Input: part model. Units: mm. Frame: model coordinates. Coordinates: 2 decimals unless noted, no trailing zeros. Loops run counter-clockwise (first coordinate to the right, second up) from the corner with the lowest first, then second, coordinate; pieces in that order, holes last. Notation, with made-up numbers: (8, 58) - (25, 58) arc R34 cw to (25, 90) - close; hole circle Ø2 at (-28, 66.5). An arc over 180 degrees is marked (long way). Use one line per item in the form item = value.
from build123d import *

# Parameters (mm, degrees)
EXTRU_MINCE1_DEPTH = 24


with BuildPart() as part:
    # Esquisse1 → Extru.-Mince1 (new body, symmetric)
    with BuildSketch(Plane.XY):
        with BuildLine():
            Line((547.565725672, -0.87294791), (541.301863245, 18.120841272))
            ThreePointArc((541.301863245, 18.120841272), (542.138161234, 23.516038085), (547, 26))
            ThreePointArc((547, 26), (551.756047412, 23.65787001), (552.799001066, 18.460004337))
            Line((552.799001066, 18.460004337), (547.665682189, -0.869999215))
            Line((547.665682189, -0.869999215), (550, -80))
            Line((550, -80), (550, -1562))
            ThreePointArc((550, -1562), (547.656854249, -1567.656854249), (542, -1570))
            Line((542, -1570), (-542, -1570))
            ThreePointArc((-542, -1570), (-547.656854249, -1567.656854249), (-550, -1562))
            Line((-550, -1562), (-550, -80))
            Line((-550, -80), (-547.665682189, -0.869999215))
            Line((-547.665682189, -0.869999215), (-552.799001066, 18.460004337))
            ThreePointArc((-552.799001066, 18.460004337), (-551.756047412, 23.65787001), (-547, 26))
            ThreePointArc((-547, 26), (-542.138161234, 23.516038085), (-541.301863245, 18.120841272))
            Line((-541.301863245, 18.120841272), (-547.565725672, -0.87294791))
            Line((-547.565725672, -0.87294791), (-544.716657295, -1.812527274))
            Line((-544.716657295, -1.812527274), (-538.452794868, 17.181261908))
            ThreePointArc((-538.452794868, 17.181261908), (-539.707241851, 25.274057128), (-547, 29))
            ThreePointArc((-547, 29), (-554.134071119, 25.486805015), (-555.698501598, 17.690006505))
            Line((-555.698501598, 17.690006505), (-550.677252807, -1.217986412))
            Line((-550.677252807, -1.217986412), (-553, -79.955759949))
            Line((-553, -79.955759949), (-553, -1562))
            ThreePointArc((-553, -1562), (-549.778174593, -1569.778174593), (-542, -1573))
            Line((-542, -1573), (542, -1573))
            ThreePointArc((542, -1573), (549.778174593, -1569.778174593), (553, -1562))
            Line((553, -1562), (553, -79.955759949))
            Line((553, -79.955759949), (550.677252807, -1.217986412))
            Line((550.677252807, -1.217986412), (555.698501598, 17.690006505))
            ThreePointArc((555.698501598, 17.690006505), (554.134071119, 25.486805015), (547, 29))
            ThreePointArc((547, 29), (539.707241851, 25.274057128), (538.452794868, 17.181261908))
            Line((538.452794868, 17.181261908), (544.716657295, -1.812527274))
            Line((544.716657295, -1.812527274), (547.565725672, -0.87294791))
        make_face()
    extrude(amount=EXTRU_MINCE1_DEPTH, both=True)


solid = part.part
Q1. Cut plane A-A, the plane y = -569. Return loops of the section in (x, z), then the cut area to 3 significant figures.
Check values:
outline = (-553, -24) - (-550, -24) - (-550, 24) - (-553, 24) - close; (550, -24) - (553, -24) - (553, 24) - (550, 24) - close
area = 288 mm²
Q2. Ray query, line 1 along X through (y, z) = (20, 9); line 2 along X through (y, z) = (-357, 6.5); line 3 along Y through (x, z) = (-143, -18.5). Return the intervals inside material, ascending. Write a range as [from, to].
Check values:
line_1 = [-556, -553], [-541, -538], [538, 541], [553, 556]
line_2 = [-553, -550], [550, 553]
line_3 = [-1573, -1570]
Q3. Pull-direction query (X, two-part tool) for faces 1 (the flat face through (-8, -1573, 0)), 2 (the flat face through (-553, -811, 0)), 3 (the flat face through (553, -831, 0)), 4 (the flat face through (-550, -831, 0)); classes: pulls with the +X half, pulls with the -X half, needs draft (parallel to the pull), parting line crosses it, or undercut.
Check values:
face_1 = needs draft
face_2 = pulls with the -X half
face_3 = pulls with the +X half
face_4 = undercut
Q4. Cut plane B-B, the plane z = -10.5. Return loops of the section in (x, y), then the cut area to 3 significant figures.
Check values:
outline = (-555.7, 17.69) - (-550.68, -1.22) - (-553, -79.96) - (-553, -1562) arc R11 ccw to (-542, -1573) - (542, -1573) arc R11 ccw to (553, -1562) - (553, -79.96) - (550.68, -1.22) - (555.7, 17.69) arc R9 ccw (long way) to (538.45, 17.18) - (544.72, -1.81) - (547.57, -0.87) - (541.3, 18.12) arc R6 cw (long way) to (552.8, 18.46) - (547.67, -0.87) - (550, -80) - (550, -1562) arc R8 cw to (542, -1570) - (-542, -1570) arc R8 cw to (-550, -1562) - (-550, -80) - (-547.67, -0.87) - (-552.8, 18.46) arc R6 cw (long way) to (-541.3, 18.12) - (-547.57, -0.87) - (-544.72, -1.81) - (-538.45, 17.18) arc R9 ccw (long way) to start
area = 13,100 mm²
Q5. First-contact query: P1, Ø12, axis at x = -375, z = -5, coming from the +Y side; P2, Ø4, axis at y = -836, z = 17.5, coming from the -X side; P3, Ø7, axis at x = 547, y = 20, coming from the +Z side; P4, Ø3, axis at y = -453, z = -5.5, coming from the +X side. Flat tips, straight axial feed; report the tip coordinate or a pass-through.
Check values:
P1 = -1570
P2 = -553
P3 = through
P4 = 553
Q6. Cut plane C-C, the plane x = -393. Return loops of the section in (y, z), then the cut area to 3 significant figures.
Check values:
outline = (-1573, -24) - (-1570, -24) - (-1570, 24) - (-1573, 24) - close
area = 144 mm²
